```python
from build123d import *

# Parameters (mm, degrees)
F0_W          = 5.7658
F0_H          = 19.8156631229
F2_R          = 4.2418
F3_DEPTH      = 19.8166631229
F5_ANGLE_BACK = 35
F5_ANGLE      = 70
F7_W          = 19.842395559
F7_H          = 3.2231725054
F8_DEPTH      = 2.54


# Not quite as in the source:
# - a feature names something its author has since deleted; it is built from what else it names


with BuildPart() as f1:
    # F0 (on Top) → F1 (revolve)
    with BuildSketch(Plane.XY):
        with Locations((2.8829, 9.9078315614)):
            Rectangle(F0_W, F0_H)
    revolve(axis=Axis((5.7658, 9.9078315614, 0), (0, -1, 0)))

    # F2 (on face) → F3 (cut, through all)
    with BuildSketch(Plane(origin=(0, 19.8156631229, 0), x_dir=(-1, 0, 0), z_dir=(0, 1, 0))):
        with Locations((-5.7658, 0)):
            Circle(F2_R)
    extrude(amount=-F3_DEPTH, mode=Mode.SUBTRACT)

    # F4 (on Top) → F5 (revolve)
    with BuildSketch(Plane.XY, mode=Mode.PRIVATE) as f5_sk:
        Polygon((0, -7.1477591426), (0, 0), (0, 3.933498799), (-1.27, 3.933498799), (-1.27, 0), (-1.27, -7.1477591426), (0, -38.1), (1.2367536547, -38.268789649), align=None)
    revolve(f5_sk.sketch.rotate(Axis((5.7658, 11.3838200413, 0), (0, -1, 0)), -F5_ANGLE_BACK), axis=Axis((5.7658, 11.3838200413, 0), (0, -1, 0)), revolution_arc=F5_ANGLE)

    # F7 (on offset) → F8 (cut)
    with BuildSketch(Plane.YZ.offset(11.7856)):
        with Locations((9.9211977795, -0.010144955)):
            Rectangle(F7_W, F7_H)
    extrude(amount=-F8_DEPTH, mode=Mode.SUBTRACT)


solid = f1.part
```
Here's how the part is built. I have some questions about the finished solid (model axes, mm). A direction names the side the tool comes from. Give positions to 0.01 mm unless a question says otherwise; leave off trailing zeros. Loops run counter-clockwise (first coordinate to the right, second up) from the corner with the lowest first, then second, coordinate; pieces in that order, holes last. Notation, with made-up numbers: (41, 53) -> (75, 53) arc R11 ccw to (75, 72) -> close; hole circle Ø11 at (25.25, -34.75). An arc over 180 degrees is marked (long way). Use one line per item in the form item = value. Start each with the question number.
1) Imagine slicing it at D-D (z = 0). Please give me the cut outline in (x, y), then the cut area to 3 significant figures.
2) Imagine slicing it at B-B (x = 8.25). Please give me the cut outline in (y, z).
3) Imagine slicing it at C-C (y = 15). Please give me the cut outline in (x, z).
4) Imagine slicing it at A-A (x = 4.75). Please give me the cut outline in (y, z), then the cut area to 3 significant figures.
5) For P1, Ø0.5, axis at x = 11, y = 5.5, coming from the +Z side; P2, Ø5, axis at y = -24.5, z = 4.5, coming from the -X side; P3, Ø1, axis at x = 1.5, y = 10, coming from the -Z side, each with a flat end and sliding along its axis, tell me the tip position at first contact or that it passes through.
6) Which directions (+Z, -Z, +X, -X, +Y, -Y) give clear straight access to the entire face, cutting with the end or side of a thin tool? Please do faces 1 (the face through (0, -4, 0)), 2 (the face through (0, 10, 0)), 3 (the face through (11, 10, -1.622)), 4 (the face through (-0.3, 3.933, -0.1)).
7) Thinking about a two-plate mould opening in Y: for faces 5 (the face through (-1.27, -1.68, 0.06)), 6 (the face through (1, 19.816, 0)), 7 (the face through (1, 0, 0)), which applies, +Y half, -Y half, draft (parallel to the pull), parting line (faces both ways), or undercut?
8) Please list where these lines run through material, in increasing order: line 1 along Y through (x, z) = (9.25, -2.5); line 2 along X through (y, z) = (7.25, 0); line 3 along Z through (x, y) = (3.25, 8).
Check values:
q1.outline = (-1.27, -7.15) -> (0, -38.1) -> (1.24, -38.27) -> (0, -7.15) -> (0, 0) -> (1.52, 0) -> (1.52, 19.82) -> (0, 19.82) -> (0, 3.93) -> (-1.27, 3.93) -> close
q1.area = 83.1 mm^2
q2.outline = (0, -5.2) -> (19.82, -5.2) -> (19.82, -3.44) -> (0, -3.44) -> close; (0, 3.44) -> (19.82, 3.44) -> (19.82, 5.2) -> (0, 5.2) -> close
q3.outline = (9.69, -1.62) arc R4.24 cw (long way) to (9.69, 1.6) -> (11.3, 1.6) arc R5.77 ccw (long way) to (11.3, -1.62) -> close
q4.outline = (0, -5.68) -> (19.82, -5.68) -> (19.82, -4.12) -> (0, -4.12) -> close; (0, 4.12) -> (19.82, 4.12) -> (19.82, 5.68) -> (0, 5.68) -> close
q4.area = 61.7 mm^2
q5.P1 = 2.9
q5.P2 = -0.24
q5.P3 = -4.37
q6.face_1 = +X
q6.face_2 = +Y
q6.face_3 = +X, +Y, -Y
q6.face_4 = -X, +Y
q7.face_5 = draft
q7.face_6 = +Y half
q7.face_7 = undercut
q8.line_1 = 0 to 19.82
q8.line_2 = 0 to 1.52
q8.line_3 = -5.19 to -3.42, 3.42 to 5.19
